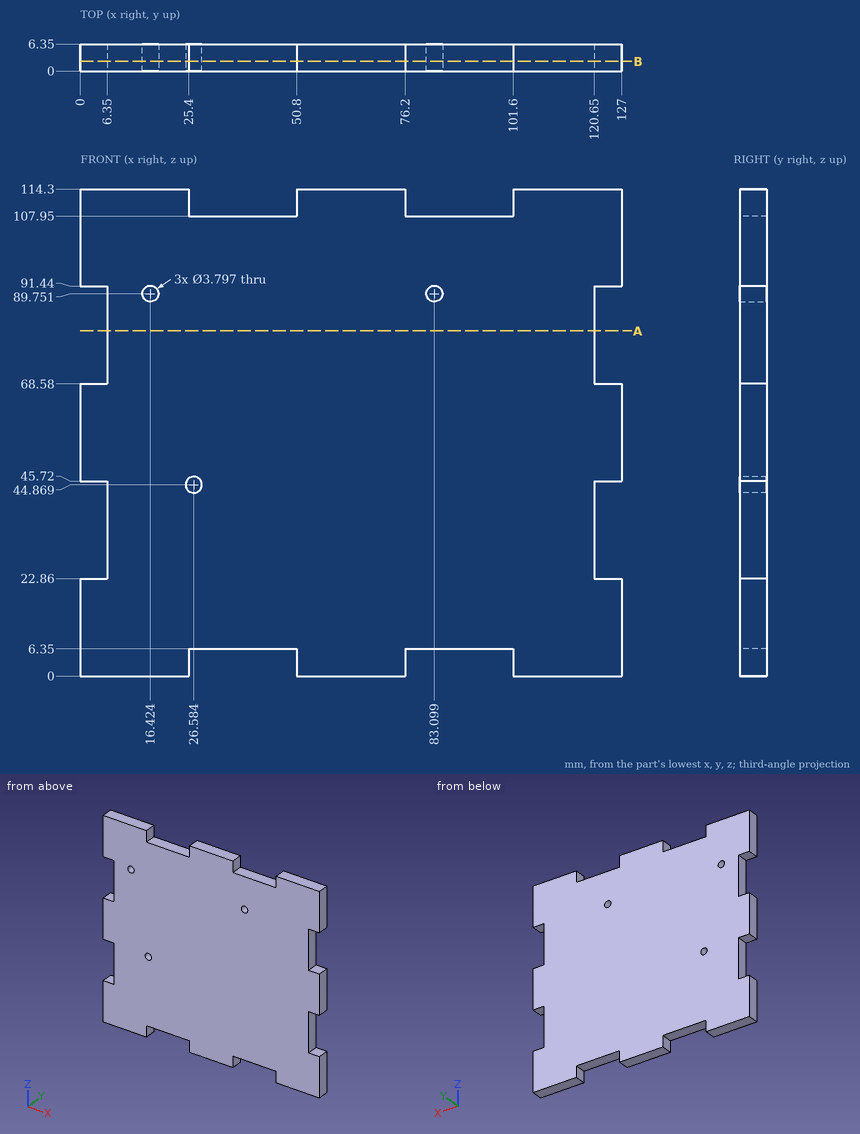
Could you check a few things on this drawing? It's one solid part, dimensions in mm from its lowest x, y, z. Give positions to 0.01 mm unless a question says otherwise; leave off trailing zeros. Write each loop counter-clockwise with the first axis right and the second up, starting at its lowest first coordinate (ties: lowest second). Pieces come first, ordered by that corner, then holes. Notation, with made-up numbers: (-20.75, 48) -> (19.25, 48) arc R18 cw to (19.25, 75) -> close; hole circle Ø9 at (-14, 55.25). An arc over 180 degrees is marked (long way). Answer as CSV lines item,"result". Start each with the question number.
(1) If we section it at A-A, the plane z = 81: Write out the boundary of the cut face in (x, y), and give its area (3 significant figures).
(2) If we section it at B-B, the plane y = 2.25: Give the number of separate pieces and of enclosed holes in the cut face, and give its area (3 significant figures).
(3) Please list where these lines run through material, in increasing order: line 1 (X direction, y = 4.25, z = 108.5); line 2 (X direction, y = 4.25, z = 29.5); line 3 (Z direction, x = 25, y = 3) (1 decimal).
(4) I'm going to push flat-ended pins straight in: pin 1 Ø2 at (y, z) = (5.5, 71.5) entering from +X; pin 2 Ø6 at (x, z) = (83.1, 89.75) entering from +Y; pin 3 Ø3 at (x, y) = (99, 1) entering from +Z. Where does each tip first touch, or does it pass through?
Answer list:
1,outline,"(6.35, 0) -> (120.65, 0) -> (120.65, 6.35) -> (6.35, 6.35) -> close"
1,area,"726 mm^2"
2,separate pieces,"1"
2,enclosed holes,"3"
2,area,"13,300 mm^2"
3,line 1,"0 to 25.4, 50.8 to 76.2, 101.6 to 127"
3,line 2,"6.35 to 120.65"
3,line 3,"0 to 43.8, 45.9 to 114.3"
4,pin 1,"x = 120.65"
4,pin 2,"y = 6.35"
4,pin 3,"z = 107.95"
